Verification items for the finished model (mm, model axes). A direction names the side the tool comes from. Give positions to 0.01 mm unless a question says otherwise; leave off trailing zeros. Order: outer loops, then holes, each group sorted by start corner. A loop starts at its lowest first (then second) coordinate and runs counter-clockwise, first axis right, second up.
(1) Scan lines: L1, parallel to Y at x = 135.5, z = -215.9 (3 decimals); L2, parallel to Z at x = 135, y = 38.1 (3 decimals); L3, parallel to Y at x = -211.75, z = -152.4 (3 decimals). Record each from-to range of solid material in increasing order.
(2) Sectioned sample at A-A on z = 130. Record the cut outline in (x, y).
(3) Mould release check, pull along Z, two halves, no side actions. Record for faces 1 (the face through (-203.2, 190, 3)), 2 (the face through (-228.6, 13, 3)): pulls with the +Z half, pulls with the -Z half, needs draft (parallel to the pull), parting line crosses it, or undercut.
(4) Gauge pin test, flat ends, axial feed: pin 1 (20.5 mm diameter, centred on y = 113, z = -213, fed in from -X); pin 2 (10 mm diameter, centred on y = 31, z = 131.5, fed in from +X); pin 3 (12.5 mm diameter, centred on y = 134.5, z = 216, fed in from +X); pin 4 (10 mm diameter, centred on y = 12.7, z = 152.4, fed in from -X). Record the tip position at first contact, or that the pin passes through.
(5) Access from +Z, -Z, +X, -X, +Y, -Y to the whole of each face (thin tool, end or side, straight path). Record for faces 3 (the face through (152.4, 101, -216)), 4 (the face through (-3, 13, -203.2)), 5 (the face through (2, 25.4, -216)), 6 (the face through (-207, 177.8, -54)), 7 (the face through (228.6, 13, 3)).
(6) Sectioned sample at B-B on y = 138. Record the cut outline in (x, z).
```python
from build123d import *

# Parameters (mm, degrees)
SKETCH1_W            = 457.2
SKETCH1_H            = 457.2
SKETCH1_W_2          = 406.4
SKETCH1_H_2          = 406.4
BOSS_EXTRUDE1_DEPTH  = 203.2
CUT_EXTRUDE3_REACH   = 552.073
SKETCH2_W            = 254
SKETCH2_H            = 152.4
SKETCH2_W_2          = 76.2
SKETCH4_W            = 215.9
SKETCH4_H            = 152.4
CUT_EXTRUDE4_DEPTH   = 25.4
SKETCH6_R            = 3.175
CUT_EXTRUDE5_DEPTH   = 25.4
CUT_EXTRUDE6_START   = -25.4
SKETCH7_R            = 3.175
CUT_EXTRUDE6_DEPTH   = 25.4
CUT_EXTRUDE7_REACH   = 552.073
SKETCH8_R            = 3.175
SKETCH10_R           = 3.175
CUT_EXTRUDE8_DEPTH   = 551.072758824
LPATTERN1_COUNT      = 2
LPATTERN1_PITCH      = 38.1
LPATTERN1_COUNT_DIR2 = 2
LPATTERN1_PITCH_DIR2 = 177.8
SKETCH12_W           = 25.4
SKETCH12_H           = 152.4
CUT_EXTRUDE9_DEPTH   = 25.4
SKETCH13_W           = 25.4
SKETCH13_H           = 152.4
BOSS_EXTRUDE2_DEPTH  = 25.4
SKETCH14_R           = 3.175
CUT_EXTRUDE11_DEPTH  = 25.4


with BuildPart() as part:
    # Sketch1 → Boss-Extrude1 (new body)
    with BuildSketch(Plane(origin=(0, 0, 0), x_dir=(1, 0, 0), z_dir=(0, 1, 0))):
        Rectangle(SKETCH1_W, SKETCH1_H)
        Rectangle(SKETCH1_W_2, SKETCH1_H_2, mode=Mode.SUBTRACT)
    extrude(amount=BOSS_EXTRUDE1_DEPTH)

    # Cut-Extrude3: up to this face of the body (flat: up to its plane)
    cut_extrude3_end = Plane(part.part.faces().sort_by_distance((0, 101.6, -203.2))[0])
    # Sketch2 → Cut-Extrude3 (cut, up to the picked face)
    with BuildSketch(Plane.XY.offset(228.6), mode=Mode.PRIVATE) as cut_extrude3_sk1:
        with Locations((0, 101.6)):
            Rectangle(SKETCH2_W, SKETCH2_H)
    cut_extrude3_tool1 = split(extrude(cut_extrude3_sk1.sketch, amount=-CUT_EXTRUDE3_REACH, mode=Mode.PRIVATE), bisect_by=cut_extrude3_end, keep=Keep.BOTH, mode=Mode.PRIVATE)
    # Sketch2 → Cut-Extrude3 (cut, up to the picked face)
    with BuildSketch(Plane.XY.offset(228.6), mode=Mode.PRIVATE) as cut_extrude3_sk2:
        with Locations((190.5, 101.6)):
            Rectangle(SKETCH2_W_2, SKETCH2_H)
    cut_extrude3_tool2 = split(extrude(cut_extrude3_sk2.sketch, amount=-CUT_EXTRUDE3_REACH, mode=Mode.PRIVATE), bisect_by=cut_extrude3_end, keep=Keep.BOTH, mode=Mode.PRIVATE)
    # Sketch2 → Cut-Extrude3 (cut, up to the picked face)
    with BuildSketch(Plane.XY.offset(228.6), mode=Mode.PRIVATE) as cut_extrude3_sk3:
        with Locations((-190.5, 101.6)):
            Rectangle(SKETCH2_W_2, SKETCH2_H)
    cut_extrude3_tool3 = split(extrude(cut_extrude3_sk3.sketch, amount=-CUT_EXTRUDE3_REACH, mode=Mode.PRIVATE), bisect_by=cut_extrude3_end, keep=Keep.BOTH, mode=Mode.PRIVATE)
    add(cut_extrude3_tool1.solids().sort_by(Axis((0, 101.6, 228.6), (0, 0, -1)))[0], mode=Mode.SUBTRACT)
    add(cut_extrude3_tool2.solids().sort_by(Axis((190.5, 101.6, 228.6), (0, 0, -1)))[0], mode=Mode.SUBTRACT)
    add(cut_extrude3_tool3.solids().sort_by(Axis((-190.5, 101.6, 228.6), (0, 0, -1)))[0], mode=Mode.SUBTRACT)

    # Sketch4 → Cut-Extrude4 (cut)
    with BuildSketch(Plane(origin=(0, 0, -228.6), x_dir=(-1, 0, 0), z_dir=(0, 0, -1))):
        with Locations((120.65, 101.6)):
            Rectangle(SKETCH4_W, SKETCH4_H)
        with Locations((-120.65, 101.6)):
            Rectangle(SKETCH4_W, SKETCH4_H)
    extrude(amount=-CUT_EXTRUDE4_DEPTH, mode=Mode.SUBTRACT)

    # Sketch6 → Cut-Extrude5 (cut)
    with BuildSketch(Plane(origin=(152.4, 0, 0), x_dir=(0, 0, -1), z_dir=(1, 0, 0))):
        with Locations(Location((-215.9, 38.1, 0), (0, 0, 90))):
            Circle(SKETCH6_R)
        with Locations(Location((-215.9, 88.9, 0), (0, 0, 90))):
            Circle(SKETCH6_R)
    extrude(amount=-CUT_EXTRUDE5_DEPTH, mode=Mode.SUBTRACT)

    # Sketch7 → Cut-Extrude6 (cut)
    with BuildSketch(Plane.ZY.offset(152.4).offset(CUT_EXTRUDE6_START)):
        with Locations((215.9, 165.1)):
            Circle(SKETCH7_R)
        with Locations((215.9, 127)):
            Circle(SKETCH7_R)
        with Locations(Location((215.9, 88.9, 0), (0, 0, 90))):
            Circle(SKETCH7_R)
    extrude(amount=CUT_EXTRUDE6_DEPTH, mode=Mode.SUBTRACT)

    # Cut-Extrude7: up to this face of the body (flat: up to its plane)
    cut_extrude7_end = Plane(part.part.faces().sort_by_distance((-228.6, 190.5, 0))[0])
    # Sketch8 → Cut-Extrude7 (cut, up to the picked face)
    with BuildSketch(Plane(origin=(228.6, 0, 0), x_dir=(0, 0, -1), z_dir=(1, 0, 0)), mode=Mode.PRIVATE) as cut_extrude7_sk1:
        with Locations((152.4, 190.5)):
            Circle(SKETCH8_R)
    cut_extrude7_tool1 = split(extrude(cut_extrude7_sk1.sketch, amount=-CUT_EXTRUDE7_REACH, mode=Mode.PRIVATE), bisect_by=cut_extrude7_end, keep=Keep.BOTH, mode=Mode.PRIVATE)
    # Sketch8 → Cut-Extrude7 (cut, up to the picked face)
    with BuildSketch(Plane(origin=(228.6, 0, 0), x_dir=(0, 0, -1), z_dir=(1, 0, 0)), mode=Mode.PRIVATE) as cut_extrude7_sk2:
        with Locations((114.3, 190.5)):
            Circle(SKETCH8_R)
    cut_extrude7_tool2 = split(extrude(cut_extrude7_sk2.sketch, amount=-CUT_EXTRUDE7_REACH, mode=Mode.PRIVATE), bisect_by=cut_extrude7_end, keep=Keep.BOTH, mode=Mode.PRIVATE)
    # Sketch8 → Cut-Extrude7 (cut, up to the picked face)
    with BuildSketch(Plane(origin=(228.6, 0, 0), x_dir=(0, 0, -1), z_dir=(1, 0, 0)), mode=Mode.PRIVATE) as cut_extrude7_sk3:
        with Locations((-152.4, 190.5)):
            Circle(SKETCH8_R)
    cut_extrude7_tool3 = split(extrude(cut_extrude7_sk3.sketch, amount=-CUT_EXTRUDE7_REACH, mode=Mode.PRIVATE), bisect_by=cut_extrude7_end, keep=Keep.BOTH, mode=Mode.PRIVATE)
    # Sketch8 → Cut-Extrude7 (cut, up to the picked face)
    with BuildSketch(Plane(origin=(228.6, 0, 0), x_dir=(0, 0, -1), z_dir=(1, 0, 0)), mode=Mode.PRIVATE) as cut_extrude7_sk4:
        with Locations((-114.3, 190.5)):
            Circle(SKETCH8_R)
    cut_extrude7_tool4 = split(extrude(cut_extrude7_sk4.sketch, amount=-CUT_EXTRUDE7_REACH, mode=Mode.PRIVATE), bisect_by=cut_extrude7_end, keep=Keep.BOTH, mode=Mode.PRIVATE)
    # Sketch8 → Cut-Extrude7 (cut, up to the picked face)
    with BuildSketch(Plane(origin=(228.6, 0, 0), x_dir=(0, 0, -1), z_dir=(1, 0, 0)), mode=Mode.PRIVATE) as cut_extrude7_sk5:
        with Locations((152.4, 12.7)):
            Circle(SKETCH8_R)
    cut_extrude7_tool5 = split(extrude(cut_extrude7_sk5.sketch, amount=-CUT_EXTRUDE7_REACH, mode=Mode.PRIVATE), bisect_by=cut_extrude7_end, keep=Keep.BOTH, mode=Mode.PRIVATE)
    # Sketch8 → Cut-Extrude7 (cut, up to the picked face)
    with BuildSketch(Plane(origin=(228.6, 0, 0), x_dir=(0, 0, -1), z_dir=(1, 0, 0)), mode=Mode.PRIVATE) as cut_extrude7_sk6:
        with Locations((114.3, 12.7)):
            Circle(SKETCH8_R)
    cut_extrude7_tool6 = split(extrude(cut_extrude7_sk6.sketch, amount=-CUT_EXTRUDE7_REACH, mode=Mode.PRIVATE), bisect_by=cut_extrude7_end, keep=Keep.BOTH, mode=Mode.PRIVATE)
    # Sketch8 → Cut-Extrude7 (cut, up to the picked face)
    with BuildSketch(Plane(origin=(228.6, 0, 0), x_dir=(0, 0, -1), z_dir=(1, 0, 0)), mode=Mode.PRIVATE) as cut_extrude7_sk7:
        with Locations((-114.3, 12.7)):
            Circle(SKETCH8_R)
    cut_extrude7_tool7 = split(extrude(cut_extrude7_sk7.sketch, amount=-CUT_EXTRUDE7_REACH, mode=Mode.PRIVATE), bisect_by=cut_extrude7_end, keep=Keep.BOTH, mode=Mode.PRIVATE)
    # Sketch8 → Cut-Extrude7 (cut, up to the picked face)
    with BuildSketch(Plane(origin=(228.6, 0, 0), x_dir=(0, 0, -1), z_dir=(1, 0, 0)), mode=Mode.PRIVATE) as cut_extrude7_sk8:
        with Locations((-152.4, 12.7)):
            Circle(SKETCH8_R)
    cut_extrude7_tool8 = split(extrude(cut_extrude7_sk8.sketch, amount=-CUT_EXTRUDE7_REACH, mode=Mode.PRIVATE), bisect_by=cut_extrude7_end, keep=Keep.BOTH, mode=Mode.PRIVATE)
    add(cut_extrude7_tool1.solids().sort_by(Axis((228.6, 190.5, -152.4), (-1, 0, 0)))[0], mode=Mode.SUBTRACT)
    add(cut_extrude7_tool2.solids().sort_by(Axis((228.6, 190.5, -114.3), (-1, 0, 0)))[0], mode=Mode.SUBTRACT)
    add(cut_extrude7_tool3.solids().sort_by(Axis((228.6, 190.5, 152.4), (-1, 0, 0)))[0], mode=Mode.SUBTRACT)
    add(cut_extrude7_tool4.solids().sort_by(Axis((228.6, 190.5, 114.3), (-1, 0, 0)))[0], mode=Mode.SUBTRACT)
    add(cut_extrude7_tool5.solids().sort_by(Axis((228.6, 12.7, -152.4), (-1, 0, 0)))[0], mode=Mode.SUBTRACT)
    add(cut_extrude7_tool6.solids().sort_by(Axis((228.6, 12.7, -114.3), (-1, 0, 0)))[0], mode=Mode.SUBTRACT)
    add(cut_extrude7_tool7.solids().sort_by(Axis((228.6, 12.7, 114.3), (-1, 0, 0)))[0], mode=Mode.SUBTRACT)
    add(cut_extrude7_tool8.solids().sort_by(Axis((228.6, 12.7, 152.4), (-1, 0, 0)))[0], mode=Mode.SUBTRACT)

    # Sketch10 → Cut-Extrude8 (cut, through all)
    with BuildSketch(Plane(origin=(228.6, 0, 0), x_dir=(0, 0, -1), z_dir=(1, 0, 0))):
        with Locations((-17.4625, 190.5)):
            Circle(SKETCH10_R)
    cut_extrude8 = extrude(amount=-CUT_EXTRUDE8_DEPTH, mode=Mode.SUBTRACT)

    # LPattern1: Cut-Extrude8 2 × 2
    with Locations(*[(0, -j * LPATTERN1_PITCH_DIR2, -i * LPATTERN1_PITCH) for i in range(LPATTERN1_COUNT) for j in range(LPATTERN1_COUNT_DIR2) if (i, j) != (0, 0)]):
        add(cut_extrude8, mode=Mode.SUBTRACT)

    # Sketch12 → Cut-Extrude9 (cut)
    with BuildSketch(Plane(origin=(0, 0, -228.6), x_dir=(-1, 0, 0), z_dir=(0, 0, -1))):
        with Locations((0, 101.6)):
            Rectangle(SKETCH12_W, SKETCH12_H)
    extrude(amount=-CUT_EXTRUDE9_DEPTH, mode=Mode.SUBTRACT)

    # Sketch13 → Boss-Extrude2 (add)
    with BuildSketch(Plane(origin=(0, 0, -228.6), x_dir=(-1, 0, 0), z_dir=(0, 0, -1))):
        with Locations((-139.7, 101.6)):
            Rectangle(SKETCH13_W, SKETCH13_H)
        with Locations((139.7, 101.6)):
            Rectangle(SKETCH13_W, SKETCH13_H)
    extrude(amount=-BOSS_EXTRUDE2_DEPTH)

    # Sketch14 → Cut-Extrude11 (cut)
    with BuildSketch(Plane.ZY.offset(-127)):
        with Locations(Location((-215.9, 127, 0), (0, 0, 359.999999316))):
            Circle(SKETCH14_R)
        with Locations(Location((-215.9, 88.9, 0), (0, 0, 359.999986507))):
            Circle(SKETCH14_R)
    extrude(amount=-CUT_EXTRUDE11_DEPTH, mode=Mode.SUBTRACT)


solid = part.part
```
Ans:
1. L1: y = 0 to 85.725, 92.075 to 123.825, 130.175 to 203.2
1. L2: z = -228.6 to -203.2, 203.2 to 212.725, 219.075 to 228.6
1. L3: y = 0 to 9.525, 15.875 to 25.4, 177.8 to 187.325, 193.675 to 203.2
2. outline: (-228.6, 0) - (-203.2, 0) - (-203.2, 25.4) - (-228.6, 25.4) - close; (-228.6, 177.8) - (-203.2, 177.8) - (-203.2, 203.2) - (-228.6, 203.2) - close; (203.2, 0) - (228.6, 0) - (228.6, 25.4) - (203.2, 25.4) - close; (203.2, 177.8) - (228.6, 177.8) - (228.6, 203.2) - (203.2, 203.2) - close
3. face 1: undercut
3. face 2: needs draft
4. pin 1: stops at x = -152.4
4. pin 2: passes through
4. pin 3: stops at x = 152.4
4. pin 4: stops at x = -228.6
5. face 3: +Z, -Z, +X
5. face 4: +Y, -Y
5. face 5: +Z, -Z
5. face 6: +Z, -Z, -X
5. face 7: +Z, -Z, +X, +Y, -Y
6. outline: (-152.4, -228.6) - (-127, -228.6) - (-127, -203.2) - (-152.4, -203.2) - close; (-152.4, 203.2) - (-127, 203.2) - (-127, 228.6) - (-152.4, 228.6) - close; (127, -228.6) - (152.4, -228.6) - (152.4, -203.2) - (127, -203.2) - close; (127, 203.2) - (152.4, 203.2) - (152.4, 228.6) - (127, 228.6) - close
